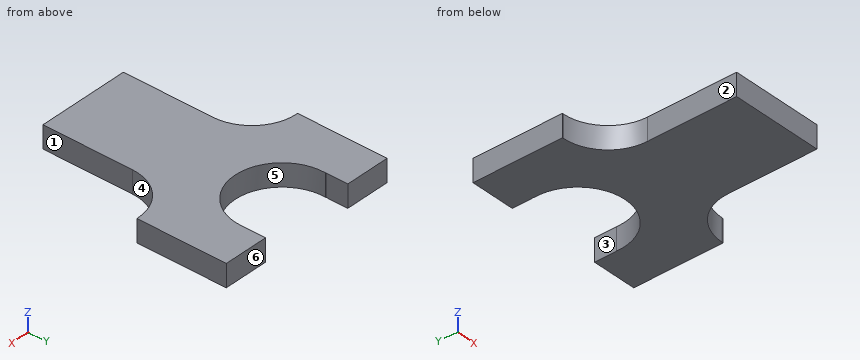
```python
from build123d import *

# Parameters (mm, degrees)
BOSS_EXTRUDE2_DEPTH = 50
CUT_EXTRUDE2_START  = -102.5
SKETCH2_R           = 3.05
CUT_EXTRUDE2_DEPTH  = 6
CUT_EXTRUDE3_START  = 96.5
SKETCH2_2_R         = 3.05
CUT_EXTRUDE3_DEPTH  = 6
BOSS_EXTRUDE3_DEPTH = 50
SKETCH5_R           = 105
CUT_EXTRUDE6_DEPTH  = 543.701575454
SKETCH8_W           = 210
SKETCH8_H           = 49.303912119
CUT_EXTRUDE7_DEPTH  = 543.701575454


with BuildPart() as part:
    # Sketch1 → Boss-Extrude2 (new body)
    with BuildSketch(Plane.XY):
        with BuildLine():
            Line((102.5, 0), (-102.5, 0))
            Line((-102.5, 0), (-102.5, 200))
            ThreePointArc((-102.5, 200), (-131.789321881, 270.710678119), (-202.5, 300))
            Line((-202.5, 300), (-205, 300))
            Line((-205, 300), (-205, 490))
            ThreePointArc((-205, 490), (-202.071067812, 497.071067812), (-195, 500))
            Line((-195, 500), (-112.5, 500))
            ThreePointArc((-112.5, 500), (-105.428932188, 497.071067812), (-102.5, 490))
            Line((-102.5, 490), (-102.5, 400.25))
            ThreePointArc((-102.5, 400.25), (-102.426776695, 400.073223305), (-102.25, 400))
            Line((-102.25, 400), (102.25, 400))
            ThreePointArc((102.25, 400), (102.426776695, 400.073223305), (102.5, 400.25))
            Line((102.5, 400.25), (102.5, 490))
            ThreePointArc((102.5, 490), (105.428932188, 497.071067812), (112.5, 500))
            Line((112.5, 500), (195, 500))
            ThreePointArc((195, 500), (202.071067812, 497.071067812), (205, 490))
            Line((205, 490), (205, 300))
            Line((205, 300), (202.5, 300))
            ThreePointArc((202.5, 300), (131.789321881, 270.710678119), (102.5, 200))
            Line((102.5, 200), (102.5, 0))
        make_face()
    extrude(amount=BOSS_EXTRUDE2_DEPTH)

    # Sketch2 → Cut-Extrude2 (cut)
    with BuildSketch(Plane(origin=(0, 0, 0), x_dir=(0, 0, -1), z_dir=(1, 0, 0)).offset(CUT_EXTRUDE2_START)):
        with Locations(Location((-25, 30, 0), (0, 0, 180))):
            Circle(SKETCH2_R)
        with Locations(Location((-25, 90, 0), (0, 0, 180))):
            Circle(SKETCH2_R)
        with Locations(Location((-25, 150, 0), (0, 0, 180))):
            Circle(SKETCH2_R)
    extrude(amount=CUT_EXTRUDE2_DEPTH, mode=Mode.SUBTRACT)

    # Sketch2<2> → Cut-Extrude3 (cut)
    with BuildSketch(Plane(origin=(0, 0, 0), x_dir=(0, 0, -1), z_dir=(1, 0, 0)).offset(CUT_EXTRUDE3_START)):
        with Locations(Location((-25, 30, 0), (0, 0, 180))):
            Circle(SKETCH2_2_R)
        with Locations(Location((-25, 90, 0), (0, 0, 180))):
            Circle(SKETCH2_2_R)
        with Locations(Location((-25, 150, 0), (0, 0, 180))):
            Circle(SKETCH2_2_R)
    extrude(amount=CUT_EXTRUDE3_DEPTH, mode=Mode.SUBTRACT)

    # Sketch6 → Boss-Extrude3 (add)
    with BuildSketch(Plane.XY):
        with BuildLine():
            Line((202.5, 300), (205, 300))
            Line((205, 300), (205, 500))
            Line((205, 500), (-205, 500))
            Line((-205, 500), (-205, 300))
            Line((-205, 300), (-202.5, 300))
            ThreePointArc((-202.5, 300), (-131.789321881, 270.710678119), (-102.5, 200))
            Line((-102.5, 200), (-102.5, 0))
            Line((-102.5, 0), (102.5, 0))
            Line((102.5, 0), (102.5, 200))
            ThreePointArc((102.5, 200), (131.789321881, 270.710678119), (202.5, 300))
        make_face()
    extrude(amount=BOSS_EXTRUDE3_DEPTH)

    # Sketch5 → Cut-Extrude6 (cut, through all)
    with BuildSketch(Plane.XY):
        with Locations((0, 445.125)):
            Circle(SKETCH5_R)
    extrude(amount=CUT_EXTRUDE6_DEPTH, mode=Mode.SUBTRACT)

    # Sketch8 → Cut-Extrude7 (cut, through all)
    with BuildSketch(Plane.XY):
        with Locations((0, 475.348043941)):
            Rectangle(SKETCH8_W, SKETCH8_H)
    extrude(amount=CUT_EXTRUDE7_DEPTH, mode=Mode.SUBTRACT)


solid = part.part
```
CAD build for the part. Positions are in the model's coordinates, mm. Face numbers are marked on the shaded views. A direction names the side the tool comes from. Round coordinates to 2 decimals unless told otherwise and drop trailing zeros. Order: outer loops, then holes, each group sorted by start corner. A loop starts at its lowest first (then second) coordinate and runs counter-clockwise, first axis right, second up.
Q1. Drop flat-ended pins along their axis: pin 1 (2 mm diameter, centred on x = -41, z = 33.5, fed in from +Y); pin 2 (8 mm diameter, centred on y = 184, z = 21, fed in from -X); pin 3 (1.2 mm diameter, centred on x = -203.5, z = 17.5, fed in from -Y). Give the stop position or say it passes through.
Q2. Wall check: L1, parallel to X at y = 478, z = 14.5; L2, parallel to X at y = 134, z = 38; L3, parallel to X at y = 221, z = 45.5. Give the ranges that are in metal, low to high.
Q3. Slice it at B-B (y = 38). Write the cut outline in (x, z).
Q4. Slice it at C-C (x = 0). Write the cut outline in (y, z) (3 decimals).
Q5. Which spindle directions (+Z, -Z, +X, -X, +Y, -Y) get a long thin tool onto all of the face, cutting with end or side? Do the marked faces 1, 2 and 3. Say none if no direction does.
Q6. Slice it at A-A (z = 30.5). Write the cut outline in (x, y) (3 decimals), and give its area (3 significant figures).
Q7. Two-plate mould, pull along X, no slides. Class the marked faces 4, 5 and 6: pulls with the +X half, pulls with the -X half, needs draft (parallel to the pull), parting line crosses it, or undercut.
Results below:
1. pin 1: stops at y = 348.89
1. pin 2: stops at x = -102.5
1. pin 3: stops at y = 300
2. L1: x = -205 to -105, 105 to 205
2. L2: x = -102.5 to 102.5
2. L3: x = -104.73 to 104.73
3. outline: (-102.5, 0) - (102.5, 0) - (102.5, 50) - (-102.5, 50) - close
4. outline: (0, 0) - (340.125, 0) - (340.125, 50) - (0, 50) - close
5. face 1: +Z, -Z, +X, -Y
5. face 2: +Z, -Z, -X, -Y
5. face 3: +Z, -Z, +Y
6. outline: (-205, 300) - (-202.5, 300) arc R100 cw to (-102.5, 200) - (-102.5, 0) - (102.5, 0) - (102.5, 200) arc R100 cw to (202.5, 300) - (205, 300) - (205, 500) - (105, 500) - (105, 450.696) - (104.852, 450.696) arc R105 cw (long way) to (-104.852, 450.696) - (-105, 450.696) - (-105, 500) - (-205, 500) - close
6. area: 119,000 mm2
7. face 4: pulls with the +X half
7. face 5: undercut
7. face 6: needs draft
